```python
from build123d import *

# Parameters (mm, degrees)
SKETCH3_R   = 36.068
SKETCH3_R_2 = 24.6253


with BuildPart() as part:
    # Sketch1 → Revolve1 (revolve)
    with BuildSketch(Plane.XY, mode=Mode.PRIVATE) as revolve1_sk:
        Polygon((-70.104, -36.068), (-31.75, -36.068), (-31.75, -30.0863), (-70.104, -30.3149), align=None)
    revolve(revolve1_sk.sketch.rotate(Axis((-70.104, 0, 0), (1, 0, 0)), 270), axis=Axis((-70.104, 0, 0), (1, 0, 0)))


with BuildPart() as body_2:
    # Sketch2 → Revolve2 (revolve)
    with BuildSketch(Plane.XY, mode=Mode.PRIVATE) as revolve2_sk:
        Polygon((30.3149, 70.104), (30.0863, 31.75), (36.068, 31.75), (36.068, 70.104), align=None)
    revolve(revolve2_sk.sketch.rotate(Axis((0, 0, 0), (0, 1, 0)), 90), axis=Axis((0, 0, 0), (0, 1, 0)))


with BuildPart() as sweep1_tool:
    # Sweep1: sweep along a path in Sketch4
    with BuildLine(Plane.XY) as sweep1_path:
        ThreePointArc((-31.75, 0), (-9.29936, 9.29936), (0, 31.75))
    # Sketch3 → Sweep1 (sweep)
    with BuildSketch(Plane(origin=(-31.75, 0, 0), x_dir=(0, 0, -1), z_dir=(1, 0, 0))):
        Circle(SKETCH3_R)
        Circle(SKETCH3_R_2, mode=Mode.SUBTRACT)
    sweep(path=sweep1_path.line)


with BuildPart() as part_1:
    add(part.part)


with BuildPart() as part_2:
    # Sweep1: joined with sweep1_tool
    add(part_1.part.fuse(sweep1_tool.part, body_2.part, tol=0.00001))


solid = part_2.part
```
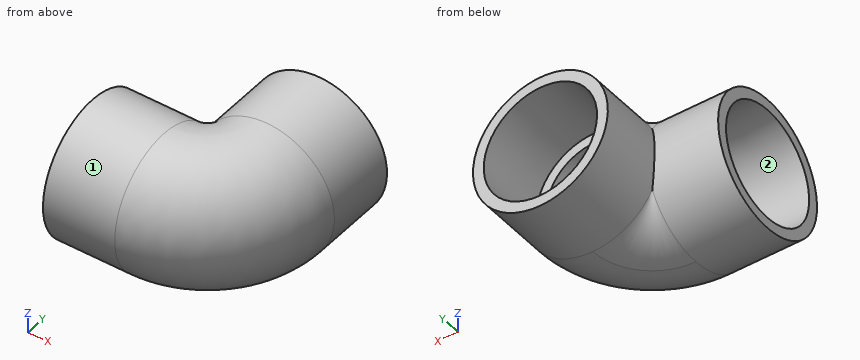
Design review of the part built by this model. Coordinates are the model's own, in mm. Face numbers are marked on the shaded views. Round coordinates to 2 decimals unless told otherwise and drop trailing zeros. Write each loop counter-clockwise with the first axis right and the second up, starting at its lowest first coordinate (ties: lowest second). Pieces come first, ordered by that corner, then holes. Notation, with made-up numbers: (-24.5, -39) -> (-3.5, -39) arc R18 ccw to (-3.5, -14) -> close; hole circle Ø8 at (9.5, 3.25). An arc over 180 degrees is marked (long way). Write item = value, one per line. Start each with the question number.
1) Wall thickness on probe 1 along Z at (x, y) = (-15.5, 5); probe 2 along Z at (x, y) = (-32, -24.5); probe 3 along X at (y, z) = (49, -24): over which ranges is each line inside the solid? List them lowest first. Write a range as from..to.
2) Mouldability with a two-part tool opening along Z and no side actions: class the marked faces 1 and 2 as +Z half, -Z half, draft (parallel to the pull), parting line (faces both ways), or undercut.
3) Take a section at A-A, the plane y = 34. State the section outline as (x, z) points.
4) Clearance check with flat-ended pins moving along their axes: pin 1 (3 mm diameter, centred on y = 54, z = -6.5, fed in from +X); pin 2 (1.5 mm diameter, centred on x = 24.5, y = 26, fed in from -Z); pin 3 (3 mm diameter, centred on x = 4.5, y = 23.5, fed in from -Z). State where each tip first meets the part, or that it passes through.
5) Take a section at B-B, the plane y = 63.5. State the section outline as (x, z) points.
Results list:
q1.probe_1 = -36.07..-24.62, 24.62..36.07
q1.probe_2 = -26.47..-17.46, 17.46..26.47
q1.probe_3 = -26.92..-18.31, 18.31..26.92
q2.face_1 = parting line
q2.face_2 = undercut
q3.outline = (-70.1, -12.04) -> (-34, -12.04) arc R36.07 ccw (long way) to (-34, 12.04) -> (-70.1, 12.04) -> close; hole circle Ø60.2 at (0, 0)
q4.pin_1 = 35.72
q4.pin_2 = -26.89
q4.pin_3 = -35.85
q5.outline = circle Ø72.14 at (0, 0); hole circle Ø60.55 at (0, 0)
